The model under review builds one solid part; all positions refer to its coordinate system, in mm. Face numbers are marked on the shaded views. A direction names the side the tool comes from. Coordinates: 2 decimals unless noted, no trailing zeros. Write each loop counter-clockwise with the first axis right and the second up, starting at its lowest first coordinate (ties: lowest second). Pieces come first, ordered by that corner, then holes. Notation, with made-up numbers: (9.25, 10.25) - (56.25, 10.25) arc R22 cw to (56.25, 41.25) - close; hole circle Ø4 at (89, -9). An arc over 180 degrees is marked (long way). Put each result on its own line as item: value. Start each with the question number.
Item 1: Consider section D-D on x = 120.5. Give the boundary of the cut face in (y, z), then the cut area to 3 significant figures.
Item 2: Consider section A-A on z = -9.5. Give the boundary of the cut face in (x, y), then the cut area to 3 significant figures.
Item 3: For pin 1 (2.5 mm diameter, centred on y = 4.5, z = -3, fed in from -X); pin 2 (6 mm diameter, centred on x = 132, y = 4.5, fed in from +Z); pin 3 (6 mm diameter, centred on x = 109.5, y = 2.5, fed in from -Z), all flat-tipped, find the tip position at first contact; note any pin that passes through.
Item 4: To check wall thickness, follow L1, parallel to Z at x = 147, y = 6.75; L2, parallel to Y at x = 150.5, z = -12.8; L3, parallel to Z at x = 241.5, y = 6. State the ranges of each line that lie inside material, in increasing order. Write a range as [from, to].
Item 5: Machinability: for the marked faces 1, 2 and 3, which of the approach directions +Z, -Z, +X, -X, +Y, -Y give a long, thin tool a straight path to every point of the face, cutting with its end or side? Answer none if there is none.
Item 6: Consider section B-B on x = 230.5. Give the boundary of the cut face in (y, z).
Item 7: Consider section C-C on y = 5. State how many separate pieces and enclosed holes the cut face has, then the cut area to 3 significant figures.
```python
from build123d import *

# Parameters (mm, degrees)
SKETCH1_W              = 250
SKETCH1_H              = 25
BOSS_EXTRUDE1_DEPTH    = 10
CUT_EXTRUDE1_REACH     = 253.446
SKETCH2_R              = 2.15
FILLET1_R              = 12.5
SKETCH3_R              = 2.25
CUT_EXTRUDE2_DEPTH     = 252.445819214
CUT_EXTRUDE5_REACH     = 253.446
SKETCH5_W              = 7.3
SKETCH5_H              = 4
SKETCH6_R              = 10
CUT_EXTRUDE6_DEPTH     = 5
CUT_EXTRUDE7_REACH     = 253.297
SKETCH7_R              = 1.65
CUT_EXTRUDE8_START     = -3.2
CUT_EXTRUDE8_OUTLINE_W = 6
CUT_EXTRUDE8_OUTLINE_H = 6
CUT_EXTRUDE8_DEPTH     = 6.4
SKETCH9_R              = 3
CUT_EXTRUDE9_DEPTH     = 2
CUT_EXTRUDE10_REACH    = 253.446
SKETCH10_W             = 60
SKETCH10_H             = 5.1
SKETCH10_W_2           = 7.3
SKETCH10_H_2           = 3.5
SKETCH11_R             = 2.25
CUT_EXTRUDE11_DEPTH    = 251.990059564


# Read off the part's stored shape, not the designer's step: Cut-Extrude8
with BuildPart() as part:
    # Sketch1 → Boss-Extrude1 (new body)
    with BuildSketch(Plane(origin=(0, 0, 0), x_dir=(1, 0, 0), z_dir=(0, 1, 0))):
        with Locations((125, 12.5)):
            Rectangle(SKETCH1_W, SKETCH1_H)
    extrude(amount=BOSS_EXTRUDE1_DEPTH)

    # Sketch2 → Cut-Extrude1 (cut, up to next)
    with BuildSketch(Plane(origin=(0, 10, 0), x_dir=(1, 0, 0), z_dir=(0, 1, 0)), mode=Mode.PRIVATE) as cut_extrude1_sk1:
        with Locations(Location((12.5, 12.5, 0), (0, 0, 270))):
            Circle(SKETCH2_R)
    cut_extrude1_tool1 = extrude(cut_extrude1_sk1.sketch, amount=-CUT_EXTRUDE1_REACH, mode=Mode.PRIVATE) & part.part
    add(cut_extrude1_tool1.solids().sort_by_distance((12.5, 10, -12.5))[0], mode=Mode.SUBTRACT)

    # Fillet1
    fillet1_edges = [part.edges().sort_by_distance(p)[0] for p in [
        (0, 5, 0),
        (0, 5, -25),
    ]]
    fillet(fillet1_edges, radius=FILLET1_R - 0.0001)  # a hair under: the kernel refuses the full size

    # Sketch3 → Cut-Extrude2 (cut, through all)
    with BuildSketch(Plane(origin=(0, 0, -25), x_dir=(-1, 0, 0), z_dir=(0, 0, -1))):
        with Locations((-244.5, 5)):
            Circle(SKETCH3_R)
        with Locations((-230.5, 5)):
            Circle(SKETCH3_R)
    extrude(amount=-CUT_EXTRUDE2_DEPTH, mode=Mode.SUBTRACT)

    # Sketch5 → Cut-Extrude5 (cut, up to next)
    with BuildSketch(Plane(origin=(0, 10, 0), x_dir=(1, 0, 0), z_dir=(0, 1, 0)), mode=Mode.PRIVATE) as cut_extrude5_sk1:
        with Locations((244.5, 19)):
            Rectangle(SKETCH5_W, SKETCH5_H)
    cut_extrude5_tool1 = extrude(cut_extrude5_sk1.sketch, amount=-CUT_EXTRUDE5_REACH, mode=Mode.PRIVATE) & part.part
    # Sketch5 → Cut-Extrude5 (cut, up to next)
    with BuildSketch(Plane(origin=(0, 10, 0), x_dir=(1, 0, 0), z_dir=(0, 1, 0)), mode=Mode.PRIVATE) as cut_extrude5_sk2:
        with Locations((244.5, 6)):
            Rectangle(SKETCH5_W, SKETCH5_H)
    cut_extrude5_tool2 = extrude(cut_extrude5_sk2.sketch, amount=-CUT_EXTRUDE5_REACH, mode=Mode.PRIVATE) & part.part
    # Sketch5 → Cut-Extrude5 (cut, up to next)
    with BuildSketch(Plane(origin=(0, 10, 0), x_dir=(1, 0, 0), z_dir=(0, 1, 0)), mode=Mode.PRIVATE) as cut_extrude5_sk3:
        with Locations((230.5, 19)):
            Rectangle(SKETCH5_W, SKETCH5_H)
    cut_extrude5_tool3 = extrude(cut_extrude5_sk3.sketch, amount=-CUT_EXTRUDE5_REACH, mode=Mode.PRIVATE) & part.part
    # Sketch5 → Cut-Extrude5 (cut, up to next)
    with BuildSketch(Plane(origin=(0, 10, 0), x_dir=(1, 0, 0), z_dir=(0, 1, 0)), mode=Mode.PRIVATE) as cut_extrude5_sk4:
        with Locations((230.5, 6)):
            Rectangle(SKETCH5_W, SKETCH5_H)
    cut_extrude5_tool4 = extrude(cut_extrude5_sk4.sketch, amount=-CUT_EXTRUDE5_REACH, mode=Mode.PRIVATE) & part.part
    add(cut_extrude5_tool1.solids().sort_by_distance((244.5, 10, -19))[0], mode=Mode.SUBTRACT)
    add(cut_extrude5_tool2.solids().sort_by_distance((244.5, 10, -6))[0], mode=Mode.SUBTRACT)
    add(cut_extrude5_tool3.solids().sort_by_distance((230.5, 10, -19))[0], mode=Mode.SUBTRACT)
    add(cut_extrude5_tool4.solids().sort_by_distance((230.5, 10, -6))[0], mode=Mode.SUBTRACT)

    # Sketch6 → Cut-Extrude6 (cut)
    with BuildSketch(Plane.XZ):
        with Locations(Location((12.5, -12.5, 0), (0, 0, 270))):
            Circle(SKETCH6_R)
    extrude(amount=-CUT_EXTRUDE6_DEPTH, mode=Mode.SUBTRACT)

    # Sketch7 → Cut-Extrude7 (cut, up to next)
    with BuildSketch(Plane.XZ.offset(-5), mode=Mode.PRIVATE) as cut_extrude7_sk1:
        with Locations(Location((12.5, -6, 0), (0, 0, 270))):
            Circle(SKETCH7_R)
    cut_extrude7_tool1 = extrude(cut_extrude7_sk1.sketch, amount=-CUT_EXTRUDE7_REACH, mode=Mode.PRIVATE) & part.part
    # Sketch7 → Cut-Extrude7 (cut, up to next)
    with BuildSketch(Plane.XZ.offset(-5), mode=Mode.PRIVATE) as cut_extrude7_sk2:
        with Locations(Location((19, -12.5, 0), (0, 0, 270))):
            Circle(SKETCH7_R)
    cut_extrude7_tool2 = extrude(cut_extrude7_sk2.sketch, amount=-CUT_EXTRUDE7_REACH, mode=Mode.PRIVATE) & part.part
    # Sketch7 → Cut-Extrude7 (cut, up to next)
    with BuildSketch(Plane.XZ.offset(-5), mode=Mode.PRIVATE) as cut_extrude7_sk3:
        with Locations(Location((12.5, -19, 0), (0, 0, 270))):
            Circle(SKETCH7_R)
    cut_extrude7_tool3 = extrude(cut_extrude7_sk3.sketch, amount=-CUT_EXTRUDE7_REACH, mode=Mode.PRIVATE) & part.part
    # Sketch7 → Cut-Extrude7 (cut, up to next)
    with BuildSketch(Plane.XZ.offset(-5), mode=Mode.PRIVATE) as cut_extrude7_sk4:
        with Locations(Location((6, -12.5, 0), (0, 0, 270))):
            Circle(SKETCH7_R)
    cut_extrude7_tool4 = extrude(cut_extrude7_sk4.sketch, amount=-CUT_EXTRUDE7_REACH, mode=Mode.PRIVATE) & part.part
    add(cut_extrude7_tool1.solids().sort_by_distance((12.5, 5, -6))[0], mode=Mode.SUBTRACT)
    add(cut_extrude7_tool2.solids().sort_by_distance((19, 5, -12.5))[0], mode=Mode.SUBTRACT)
    add(cut_extrude7_tool3.solids().sort_by_distance((12.5, 5, -19))[0], mode=Mode.SUBTRACT)
    add(cut_extrude7_tool4.solids().sort_by_distance((6, 5, -12.5))[0], mode=Mode.SUBTRACT)

    # Cut-Extrude8 outline → Cut-Extrude8 (cut)
    with BuildSketch(Plane(origin=(0, 0, 0), x_dir=(0.707106781186548, 0, -0.707106781186547), z_dir=(0.707106781186547, 0, 0.707106781186548)).offset(CUT_EXTRUDE8_START)):
        with Locations((7, 2)):
            Rectangle(CUT_EXTRUDE8_OUTLINE_W, CUT_EXTRUDE8_OUTLINE_H)
    extrude(amount=CUT_EXTRUDE8_DEPTH, mode=Mode.SUBTRACT)

    # Sketch9 → Cut-Extrude9 (cut)
    with BuildSketch(Plane(origin=(0, 10, 0), x_dir=(1, 0, 0), z_dir=(0, 1, 0))):
        with Locations(Location((12.5, 19, 0), (0, 0, 270))):
            Circle(SKETCH9_R)
        with Locations(Location((19, 12.5, 0), (0, 0, 270))):
            Circle(SKETCH9_R)
        with Locations(Location((12.5, 6, 0), (0, 0, 270))):
            Circle(SKETCH9_R)
        with Locations(Location((6, 12.5, 0), (0, 0, 270))):
            Circle(SKETCH9_R)
    extrude(amount=-CUT_EXTRUDE9_DEPTH, mode=Mode.SUBTRACT)

    # Sketch10 → Cut-Extrude10 (cut, up to next)
    with BuildSketch(Plane(origin=(0, 10, 0), x_dir=(1, 0, 0), z_dir=(0, 1, 0)), mode=Mode.PRIVATE) as cut_extrude10_sk1:
        Polygon((0, 25), (0, 0), (96, 0), (96, 5.1), (96, 19.9), (96, 25), align=None)
    cut_extrude10_tool1 = extrude(cut_extrude10_sk1.sketch, amount=-CUT_EXTRUDE10_REACH, mode=Mode.PRIVATE) & part.part
    # Sketch10 → Cut-Extrude10 (cut, up to next)
    with BuildSketch(Plane(origin=(0, 10, 0), x_dir=(1, 0, 0), z_dir=(0, 1, 0)), mode=Mode.PRIVATE) as cut_extrude10_sk2:
        with Locations((126, 2.55)):
            Rectangle(SKETCH10_W, SKETCH10_H)
    cut_extrude10_tool2 = extrude(cut_extrude10_sk2.sketch, amount=-CUT_EXTRUDE10_REACH, mode=Mode.PRIVATE) & part.part
    # Sketch10 → Cut-Extrude10 (cut, up to next)
    with BuildSketch(Plane(origin=(0, 10, 0), x_dir=(1, 0, 0), z_dir=(0, 1, 0)), mode=Mode.PRIVATE) as cut_extrude10_sk3:
        with Locations((126, 22.45)):
            Rectangle(SKETCH10_W, SKETCH10_H)
    cut_extrude10_tool3 = extrude(cut_extrude10_sk3.sketch, amount=-CUT_EXTRUDE10_REACH, mode=Mode.PRIVATE) & part.part
    # Sketch10 → Cut-Extrude10 (cut, up to next)
    with BuildSketch(Plane(origin=(0, 10, 0), x_dir=(1, 0, 0), z_dir=(0, 1, 0)), mode=Mode.PRIVATE) as cut_extrude10_sk4:
        with Locations((140.5, 15.65)):
            Rectangle(SKETCH10_W_2, SKETCH10_H_2)
    cut_extrude10_tool4 = extrude(cut_extrude10_sk4.sketch, amount=-CUT_EXTRUDE10_REACH, mode=Mode.PRIVATE) & part.part
    # Sketch10 → Cut-Extrude10 (cut, up to next)
    with BuildSketch(Plane(origin=(0, 10, 0), x_dir=(1, 0, 0), z_dir=(0, 1, 0)), mode=Mode.PRIVATE) as cut_extrude10_sk5:
        with Locations((150.5, 15.65)):
            Rectangle(SKETCH10_W_2, SKETCH10_H_2)
    cut_extrude10_tool5 = extrude(cut_extrude10_sk5.sketch, amount=-CUT_EXTRUDE10_REACH, mode=Mode.PRIVATE) & part.part
    # Sketch10 → Cut-Extrude10 (cut, up to next)
    with BuildSketch(Plane(origin=(0, 10, 0), x_dir=(1, 0, 0), z_dir=(0, 1, 0)), mode=Mode.PRIVATE) as cut_extrude10_sk6:
        with Locations((130.5, 15.65)):
            Rectangle(SKETCH10_W_2, SKETCH10_H_2)
    cut_extrude10_tool6 = extrude(cut_extrude10_sk6.sketch, amount=-CUT_EXTRUDE10_REACH, mode=Mode.PRIVATE) & part.part
    # Sketch10 → Cut-Extrude10 (cut, up to next)
    with BuildSketch(Plane(origin=(0, 10, 0), x_dir=(1, 0, 0), z_dir=(0, 1, 0)), mode=Mode.PRIVATE) as cut_extrude10_sk7:
        with Locations((120.5, 15.65)):
            Rectangle(SKETCH10_W_2, SKETCH10_H_2)
    cut_extrude10_tool7 = extrude(cut_extrude10_sk7.sketch, amount=-CUT_EXTRUDE10_REACH, mode=Mode.PRIVATE) & part.part
    # Sketch10 → Cut-Extrude10 (cut, up to next)
    with BuildSketch(Plane(origin=(0, 10, 0), x_dir=(1, 0, 0), z_dir=(0, 1, 0)), mode=Mode.PRIVATE) as cut_extrude10_sk8:
        with Locations((110.5, 15.65)):
            Rectangle(SKETCH10_W_2, SKETCH10_H_2)
    cut_extrude10_tool8 = extrude(cut_extrude10_sk8.sketch, amount=-CUT_EXTRUDE10_REACH, mode=Mode.PRIVATE) & part.part
    # Sketch10 → Cut-Extrude10 (cut, up to next)
    with BuildSketch(Plane(origin=(0, 10, 0), x_dir=(1, 0, 0), z_dir=(0, 1, 0)), mode=Mode.PRIVATE) as cut_extrude10_sk9:
        with Locations((150.5, 9.35)):
            Rectangle(SKETCH10_W_2, SKETCH10_H_2)
    cut_extrude10_tool9 = extrude(cut_extrude10_sk9.sketch, amount=-CUT_EXTRUDE10_REACH, mode=Mode.PRIVATE) & part.part
    # Sketch10 → Cut-Extrude10 (cut, up to next)
    with BuildSketch(Plane(origin=(0, 10, 0), x_dir=(1, 0, 0), z_dir=(0, 1, 0)), mode=Mode.PRIVATE) as cut_extrude10_sk10:
        with Locations((140.5, 9.35)):
            Rectangle(SKETCH10_W_2, SKETCH10_H_2)
    cut_extrude10_tool10 = extrude(cut_extrude10_sk10.sketch, amount=-CUT_EXTRUDE10_REACH, mode=Mode.PRIVATE) & part.part
    # Sketch10 → Cut-Extrude10 (cut, up to next)
    with BuildSketch(Plane(origin=(0, 10, 0), x_dir=(1, 0, 0), z_dir=(0, 1, 0)), mode=Mode.PRIVATE) as cut_extrude10_sk11:
        with Locations((130.5, 9.35)):
            Rectangle(SKETCH10_W_2, SKETCH10_H_2)
    cut_extrude10_tool11 = extrude(cut_extrude10_sk11.sketch, amount=-CUT_EXTRUDE10_REACH, mode=Mode.PRIVATE) & part.part
    # Sketch10 → Cut-Extrude10 (cut, up to next)
    with BuildSketch(Plane(origin=(0, 10, 0), x_dir=(1, 0, 0), z_dir=(0, 1, 0)), mode=Mode.PRIVATE) as cut_extrude10_sk12:
        with Locations((120.5, 9.35)):
            Rectangle(SKETCH10_W_2, SKETCH10_H_2)
    cut_extrude10_tool12 = extrude(cut_extrude10_sk12.sketch, amount=-CUT_EXTRUDE10_REACH, mode=Mode.PRIVATE) & part.part
    # Sketch10 → Cut-Extrude10 (cut, up to next)
    with BuildSketch(Plane(origin=(0, 10, 0), x_dir=(1, 0, 0), z_dir=(0, 1, 0)), mode=Mode.PRIVATE) as cut_extrude10_sk13:
        with Locations((110.5, 9.35)):
            Rectangle(SKETCH10_W_2, SKETCH10_H_2)
    cut_extrude10_tool13 = extrude(cut_extrude10_sk13.sketch, amount=-CUT_EXTRUDE10_REACH, mode=Mode.PRIVATE) & part.part
    add(cut_extrude10_tool1.solids().sort_by_distance((48, 10, -12.5))[0], mode=Mode.SUBTRACT)
    add(cut_extrude10_tool2.solids().sort_by_distance((126, 10, -2.55))[0], mode=Mode.SUBTRACT)
    add(cut_extrude10_tool3.solids().sort_by_distance((126, 10, -22.45))[0], mode=Mode.SUBTRACT)
    add(cut_extrude10_tool4.solids().sort_by_distance((140.5, 10, -15.65))[0], mode=Mode.SUBTRACT)
    add(cut_extrude10_tool5.solids().sort_by_distance((150.5, 10, -15.65))[0], mode=Mode.SUBTRACT)
    add(cut_extrude10_tool6.solids().sort_by_distance((130.5, 10, -15.65))[0], mode=Mode.SUBTRACT)
    add(cut_extrude10_tool7.solids().sort_by_distance((120.5, 10, -15.65))[0], mode=Mode.SUBTRACT)
    add(cut_extrude10_tool8.solids().sort_by_distance((110.5, 10, -15.65))[0], mode=Mode.SUBTRACT)
    add(cut_extrude10_tool9.solids().sort_by_distance((150.5, 10, -9.35))[0], mode=Mode.SUBTRACT)
    add(cut_extrude10_tool10.solids().sort_by_distance((140.5, 10, -9.35))[0], mode=Mode.SUBTRACT)
    add(cut_extrude10_tool11.solids().sort_by_distance((130.5, 10, -9.35))[0], mode=Mode.SUBTRACT)
    add(cut_extrude10_tool12.solids().sort_by_distance((120.5, 10, -9.35))[0], mode=Mode.SUBTRACT)
    add(cut_extrude10_tool13.solids().sort_by_distance((110.5, 10, -9.35))[0], mode=Mode.SUBTRACT)

    # Sketch11 → Cut-Extrude11 (cut, through all)
    with BuildSketch(Plane(origin=(0, 0, -19.9), x_dir=(-1, 0, 0), z_dir=(0, 0, -1))):
        with Locations((-150.5, 5)):
            Circle(SKETCH11_R)
        with Locations(Location((-140.5, 5, 0), (0, 0, 180))):
            Circle(SKETCH11_R)
        with Locations((-130.5, 5)):
            Circle(SKETCH11_R)
        with Locations(Location((-120.5, 5, 0), (0, 0, 180))):
            Circle(SKETCH11_R)
        with Locations(Location((-110.5, 5, 0), (0, 0, 180))):
            Circle(SKETCH11_R)
    extrude(amount=-CUT_EXTRUDE11_DEPTH, mode=Mode.SUBTRACT)


solid = part.part
```
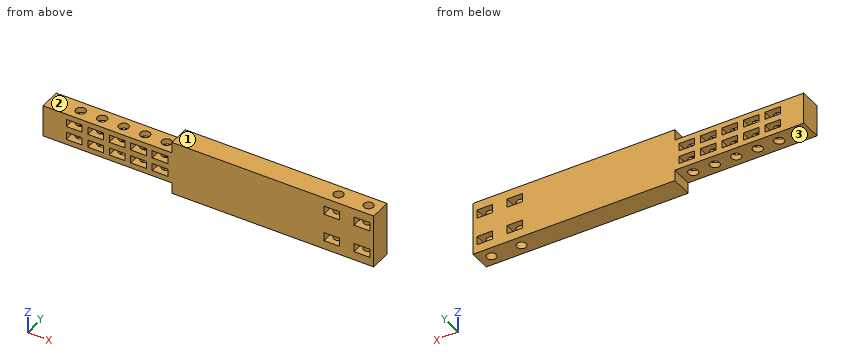
Report:
1. outline: (0, -19.9) - (2.75, -19.9) - (2.75, -17.4) - (0, -17.4) - close; (0, -13.9) - (2.75, -13.9) - (2.75, -11.1) - (0, -11.1) - close; (0, -7.6) - (2.75, -7.6) - (2.75, -5.1) - (0, -5.1) - close; (7.25, -19.9) - (10, -19.9) - (10, -17.4) - (7.25, -17.4) - close; (7.25, -13.9) - (10, -13.9) - (10, -11.1) - (7.25, -11.1) - close; (7.25, -7.6) - (10, -7.6) - (10, -5.1) - (7.25, -5.1) - close
1. area: 42.9 mm²
2. outline: (96, 0) - (106.85, 0) - (106.85, 10) - (96, 10) - close; (114.15, 0) - (116.85, 0) - (116.85, 10) - (114.15, 10) - close; (124.15, 0) - (126.85, 0) - (126.85, 10) - (124.15, 10) - close; (134.15, 0) - (136.85, 0) - (136.85, 10) - (134.15, 10) - close; (144.15, 0) - (146.85, 0) - (146.85, 10) - (144.15, 10) - close; (154.15, 0) - (250, 0) - (250, 10) - (154.15, 10) - close; hole circle Ø4.5 at (230.5, 5); hole circle Ø4.5 at (244.5, 5)
2. area: 1,140 mm²
3. pin 1: x = 156
3. pin 2: z = -5.1
3. pin 3: z = -19.9
4. L1: [-19.9, -17.4], [-13.9, -11.1], [-7.6, -5.1]
4. L2: [0, 2.75], [7.25, 10]
4. L3: [-25, -21], [-17, -8], [-4, 0]
5. face 1: +Z, +X, -X, +Y, -Y
5. face 2: +Z, -X, +Y, -Y
5. face 3: -Z, -X, +Y, -Y
6. outline: (0, -25) - (2.75, -25) - (2.75, -21) - (0, -21) - close; (0, -17) - (2.75, -17) - (2.75, -8) - (0, -8) - close; (0, -4) - (2.75, -4) - (2.75, 0) - (0, 0) - close; (7.25, -25) - (10, -25) - (10, -21) - (7.25, -21) - close; (7.25, -17) - (10, -17) - (10, -8) - (7.25, -8) - close; (7.25, -4) - (10, -4) - (10, 0) - (7.25, 0) - close
7. separate pieces: 8
7. enclosed holes: 0
7. area: 2,540 mm²
